The listing builds one solid part. Answer for the finished solid, in the listing's coordinates (mm). A direction names the side the tool comes from. Coordinates: 2 decimals unless noted, no trailing zeros. Loops run counter-clockwise (first coordinate to the right, second up) from the corner with the lowest first, then second, coordinate; pieces in that order, holes last. Notation, with made-up numbers: (18, -29) - (72, -29) arc R22 cw to (72, 4) - close; hole circle Ø11 at (57, 55.5). An arc over 180 degrees is marked (long way). Return JSON: item names as keys, results as strings. Group by question number.
1. Section D-D (z = -5.25) is taken. Write down the section's boundary in (x, y), and give its area (3 significant figures).
2. Section B-B (z = -2.25) is taken. Write down the section's boundary in (x, y), and give its area (3 significant figures).
3. Each of these flat-tipped pins is pushed along its axis until it touches: P1, Ø6, axis at x = 59.5, y = -20.5, coming from the -Z side; P2, Ø3, axis at y = 1, z = -2, coming from the -X side; P3, Ø1, axis at x = 59.5, z = -2.5, coming from the +Y side. Where does it stop, or does it pass through?
4. The mould has two halves that part along X. Classify faces 4 (the face through (62.512, 21.685, -0.592)), 5 (the face through (11.7, -25, -2)), 6 (the face through (56.424, 0.264, -3.938)): pulls with the +X half, pulls with the -X half, needs draft (parallel to the pull), parting line crosses it, or undercut.
5. Find the intervals of material crossed by line 1 along Y through (x, z) = (43.5, -2.5); line 2 along Y through (x, z) = (50.43, -5.85); line 3 along Y through (x, z) = (46, -1.5), in increasing order.
6. Which of the six approach directions +Z, -Z, +X, -X, +Y, -Y give full straight-line access (tool end or side, diameter ignored) to faces 1 (the face through (29, 23.6, -2)), 2 (the face through (67, 0, -1.2)), 3 (the face through (60.511, -19.706, -2.186))?
```python
from build123d import *

# Parameters (mm, degrees)
SKETCH_2_R            = 2.6
EXTRUDE_1_DEPTH       = 1.2
EXTRUDE_1_2_DEPTH     = 2
CUT_EXTRUDE_START     = -2
CUT_EXTRUDE_1_DEPTH   = 2
SKETCH_7_W            = 2
SKETCH_7_H            = 51.2
EXTRUDE_2_DEPTH       = 0.4
SKETCH_8_W            = 2.4
SKETCH_8_H            = 47.2
CUT_EXTRUDE_1_2_DEPTH = 2
CUT_EXTRUDE_2_DEPTH   = 62
SKETCH_10_W           = 2
SKETCH_10_H           = 2
CUT_EXTRUDE_3_DEPTH   = 0.2
SKETCH_11_W           = 14.43
SKETCH_11_H           = 14
SKETCH_11_R           = 2.6
EXTRUDE_3_DEPTH       = 5.4
SKETCH_12_R           = 3
SKETCH_12_R_2         = 2
EXTRUDE_2_2_DEPTH     = 2
SKETCH_13_R           = 3.1
CUT_EXTRUDE_4_DEPTH   = 4.6
CHAMFER_1_SIZE        = 1.1
SKETCH_14_R           = 11
SKETCH_14_R_2         = 6
CUT_EXTRUDE_2_2_DEPTH = 5.4


with BuildPart() as part:
    # Эскиз2 → Extrude 1 (new body)
    with BuildSketch(Plane.XY):
        with BuildLine():
            Line((68.5, -7), (68.5, 7))
            ThreePointArc((68.5, 7), (62.349242405, 21.849242405), (47.5, 28))
            Line((47.5, 28), (11.5, 28))
            Line((11.5, 28), (11.5, -28))
            Line((11.5, -28), (47.5, -28))
            ThreePointArc((47.5, -28), (62.349242405, -21.849242405), (68.5, -7))
        make_face()
        with Locations((50.43, 0)):
            Circle(SKETCH_2_R, mode=Mode.SUBTRACT)
    extrude(amount=-EXTRUDE_1_DEPTH)

    # Эскиз3 → Extrude 1 2 (add)
    with BuildSketch(Plane(origin=(0, 0, -1.2), x_dir=(-1, 0, 0), z_dir=(0, 0, -1))):
        with BuildLine():
            Line((-46.5, -26), (-11.5, -26))
            Line((-11.5, -26), (-11.5, 26))
            Line((-11.5, 26), (-46.5, 26))
            ThreePointArc((-46.5, 26), (-60.642135624, 20.142135624), (-66.5, 6))
            Line((-66.5, 6), (-66.5, -6))
            ThreePointArc((-66.5, -6), (-60.642135624, -20.142135624), (-46.5, -26))
        make_face()
        with BuildLine():
            Line((-46.5, -23.6), (-13.9, -23.6))
            Line((-13.9, -23.6), (-13.9, 23.6))
            Line((-13.9, 23.6), (-46.5, 23.6))
            ThreePointArc((-46.5, 23.6), (-58.945079349, 18.445079349), (-64.1, 6))
            Line((-64.1, 6), (-64.1, -6))
            ThreePointArc((-64.1, -6), (-58.945079349, -18.445079349), (-46.5, -23.6))
        make_face(mode=Mode.SUBTRACT)
    extrude(amount=EXTRUDE_1_2_DEPTH)

    # Эскиз4 → Cut-Extrude 1 (cut)
    with BuildSketch(Plane(origin=(0, 0, -3.2), x_dir=(-1, 0, 0), z_dir=(0, 0, -1)).offset(CUT_EXTRUDE_START)):
        with BuildLine():
            Line((-66.5, 6), (-66.5, -6))
            ThreePointArc((-66.5, -6), (-60.642135624, -20.142135624), (-46.5, -26))
            Line((-46.5, -26), (-11.5, -26))
            Line((-11.5, -26), (-11.5, 26))
            Line((-11.5, 26), (-46.5, 26))
            ThreePointArc((-46.5, 26), (-60.642135624, 20.142135624), (-66.5, 6))
        make_face()
        with BuildLine():
            Line((-66.1, 6), (-66.1, -6))
            ThreePointArc((-66.1, -6), (-60.359292911, -19.859292911), (-46.5, -25.6))
            Line((-46.5, -25.6), (-11.9, -25.6))
            Line((-11.9, -25.6), (-11.9, 25.6))
            Line((-11.9, 25.6), (-46.5, 25.6))
            ThreePointArc((-46.5, 25.6), (-60.359292911, 19.859292911), (-66.1, 6))
        make_face(mode=Mode.SUBTRACT)
    extrude(amount=CUT_EXTRUDE_1_DEPTH, mode=Mode.SUBTRACT)

    # Эскиз7 → Extrude 2 (add)
    with BuildSketch(Plane.ZY.offset(-11.9)):
        with Locations((-2.2, 0)):
            Rectangle(SKETCH_7_W, SKETCH_7_H)
    extrude(amount=EXTRUDE_2_DEPTH)

    # Эскиз8 → Cut-Extrude 1 2 (cut)
    with BuildSketch(Plane(origin=(0, 0, -3.2), x_dir=(-1, 0, 0), z_dir=(0, 0, -1))):
        with Locations((-12.7, 0)):
            Rectangle(SKETCH_8_W, SKETCH_8_H)
    extrude(amount=-CUT_EXTRUDE_1_2_DEPTH, mode=Mode.SUBTRACT)

    # Эскиз9 → Cut-Extrude 2 (cut)
    with BuildSketch(Plane(origin=(0, 28, 0), x_dir=(1, 0, 0), z_dir=(0, 1, 0))):
        Polygon((11.5, 0), (12.9, 0), (11.7, 1.2), (11.5, 1.2), align=None)
    extrude(amount=-CUT_EXTRUDE_2_DEPTH, mode=Mode.SUBTRACT)

    # Эскиз10 → Вырез-Вытянуть3 (cut)
    with BuildSketch(Plane.ZY.offset(-11.5)):
        with Locations((-2.2, 24.6)):
            Rectangle(SKETCH_10_W, SKETCH_10_H)
        with Locations((-2.2, -24.6)):
            Rectangle(SKETCH_10_W, SKETCH_10_H)
    extrude(amount=-CUT_EXTRUDE_3_DEPTH, mode=Mode.SUBTRACT)

    # Эскиз11 → Бобышка-Вытянуть3 (add)
    with BuildSketch(Plane(origin=(0, 0, -1.2), x_dir=(-1, 0, 0), z_dir=(0, 0, -1))):
        with Locations((-50.215, 0)):
            Rectangle(SKETCH_11_W, SKETCH_11_H)
        with Locations(Location((-50.43, 0, 0), (0, 0, 180))):
            Circle(SKETCH_11_R, mode=Mode.SUBTRACT)
    extrude(amount=EXTRUDE_3_DEPTH)

    # Эскиз12 → Extrude 2 2 (add)
    with BuildSketch(Plane(origin=(0, 0, -6.6), x_dir=(-1, 0, 0), z_dir=(0, 0, -1))):
        with Locations((-50.43, 0)):
            Circle(SKETCH_12_R)
        with Locations((-50.43, 0)):
            Circle(SKETCH_12_R_2, mode=Mode.SUBTRACT)
    extrude(amount=-EXTRUDE_2_2_DEPTH)

    # Эскиз13 → Вырез-Вытянуть4 (cut)
    with BuildSketch(Plane.XY):
        with Locations((50.43, 0)):
            Circle(SKETCH_13_R)
    extrude(amount=-CUT_EXTRUDE_4_DEPTH, mode=Mode.SUBTRACT)

    # Фаска1
    chamfer_1_edges = [part.edges().sort_by_distance(p)[0] for p in [
        (47.33, 0, -4.6),
    ]]
    chamfer(chamfer_1_edges, length=CHAMFER_1_SIZE - 0.0001)  # a hair under: the kernel refuses the full size

    # Эскиз14 → Cut-Extrude 2 2 (cut)
    with BuildSketch(Plane(origin=(0, 0, -6.6), x_dir=(-1, 0, 0), z_dir=(0, 0, -1))):
        with Locations((-50.43, 0)):
            Circle(SKETCH_14_R)
        with Locations((-50.43, 0)):
            Circle(SKETCH_14_R_2, mode=Mode.SUBTRACT)
    extrude(amount=-CUT_EXTRUDE_2_2_DEPTH, mode=Mode.SUBTRACT)


solid = part.part
```
The answers:
{
 "1": {"outline": "circle Ø12 at (50.43, 0); hole circle Ø4 at (50.43, 0)", "area": "101 mm2"},
 "2": {"outline": "(11.7, -25.6) - (46.5, -25.6) arc R19.6 ccw to (66.1, -6) - (66.1, 6) arc R19.6 ccw to (46.5, 25.6) - (11.7, 25.6) - (11.7, 23.6) - (46.5, 23.6) arc R17.6 cw to (64.1, 6) - (64.1, -6) arc R17.6 cw to (46.5, -23.6) - (11.7, -23.6) - close; circle Ø12 at (50.43, 0); hole circle Ø6.2 at (50.43, 0)", "area": "363 mm2"},
 "3": {"P1": "stops at z = -3.2", "P2": "stops at x = 11.7", "P3": "stops at y = 21.1"},
 "4": {"face 4": "pulls with the +X half", "face 5": "pulls with the -X half", "face 6": "undercut"},
 "5": {"line 1": "y = -25.6 to -23.6, 23.6 to 25.6", "line 2": "y = -6 to -2, 2 to 6", "line 3": "y = -25.6 to -23.6, -4.05 to 4.05, 23.6 to 25.6"},
 "6": {"face 1": "-Z, -X", "face 2": "-Z, +X", "face 3": "-Z, +X, -Y"}
}
